For this review, take the finished solid that the model builds, in its own axes (mm). A direction names the side the tool comes from. Round coordinates to 2 decimals unless told otherwise and drop trailing zeros. Loops run counter-clockwise (first coordinate to the right, second up) from the corner with the lowest first, then second, coordinate; pieces in that order, holes last. Notation, with made-up numbers: M 76.25,-39.5 L 85.25,-39.5 A15 ccw 85.25,-17.5 Z; hole C 39.25,42 d6. An arc over 180 degrees is marked long. Write item = value, one per line. Start each with the question number.
```python
from build123d import *

# Parameters (mm, degrees)
SKETCH1_W          = 101.6
SKETCH1_H          = 101.6
EXTRUDE1_DEPTH     = 79.502
SKETCH2_R          = 33.401
EXTRUDE2_DEPTH     = 9.398
CHAMFER1_SIZE      = 1.524
SKETCH3_R          = 13.4874
CUT_EXTRUDE1_DEPTH = 89.9
EXTRUDE3_DEPTH     = 16.002
CHAMFER2_SIZE      = 25.4
SKETCH8_R          = 5.5499
CUT_EXTRUDE3_DEPTH = 12.7


with BuildPart() as part:
    # Sketch1 → Extrude1 (new body)
    with BuildSketch(Plane(origin=(0, 0, 0), x_dir=(1, 0, 0), z_dir=(0, 1, 0))):
        Rectangle(SKETCH1_W, SKETCH1_H)
    extrude(amount=EXTRUDE1_DEPTH)

    # Sketch2 → Extrude2 (add)
    with BuildSketch(Plane(origin=(0, 79.502, 0), x_dir=(-1, 0, 0), z_dir=(0, 1, 0))):
        with Locations(Location((0, 0, 0), (0, 0, 90))):  # turned: the seam where the file's is
            Circle(SKETCH2_R)
    extrude(amount=EXTRUDE2_DEPTH)

    # Chamfer1
    chamfer1_edges = [part.edges().sort_by_distance(p)[0] for p in [
        (0, 88.9, -33.401),
    ]]
    chamfer(chamfer1_edges, length=CHAMFER1_SIZE)

    # Sketch3 → Cut-Extrude1 (cut, through all)
    with BuildSketch(Plane(origin=(0, 88.9, 0), x_dir=(1, 0, 0), z_dir=(0, 1, 0))):
        with Locations(Location((0, 0, 0), (0, 0, 270))):  # turned: the seam where the file's is
            Circle(SKETCH3_R)
    extrude(amount=-CUT_EXTRUDE1_DEPTH, mode=Mode.SUBTRACT)

    # Sketch7 → Extrude3 (add)
    with BuildSketch(Plane.XZ):
        with BuildLine():
            Line((50.8, 50.8), (82.55, 50.8))
            Line((82.55, 50.8), (82.55, 6.731))
            Line((82.55, 6.731), (63.5, 6.731))
            ThreePointArc((63.5, 6.731), (56.769, 0), (63.5, -6.731))
            Line((63.5, -6.731), (82.55, -6.731))
            Line((82.55, -6.731), (82.55, -50.8))
            Line((82.55, -50.8), (50.8, -50.8))
            Line((50.8, -50.8), (50.8, 50.8))
        make_face()
        with BuildLine():
            Line((-82.55, -6.731), (-82.55, -50.8))
            Line((-82.55, -50.8), (-50.8, -50.8))
            Line((-50.8, -50.8), (-50.8, 50.8))
            Line((-50.8, 50.8), (-82.55, 50.8))
            Line((-82.55, 50.8), (-82.55, 6.731))
            Line((-82.55, 6.731), (-63.5, 6.731))
            ThreePointArc((-63.5, 6.731), (-56.769, 0), (-63.5, -6.731))
            Line((-63.5, -6.731), (-82.55, -6.731))
        make_face()
    extrude(amount=-EXTRUDE3_DEPTH)

    # Chamfer2
    chamfer2_edges = [part.edges().sort_by_distance(p)[0] for p in [
        (-82.55, 8.001, -50.8),
        (82.55, 8.001, -50.8),
        (82.55, 8.001, 50.8),
        (-82.55, 8.001, 50.8),
    ]]
    chamfer(chamfer2_edges, length=CHAMFER2_SIZE)

    # Sketch8 → Cut-Extrude3 (cut)
    with BuildSketch(Plane.XY.offset(50.8)):
        with Locations((0, 69.85)):
            Circle(SKETCH8_R)
        with Locations((0, 12.7)):
            Circle(SKETCH8_R)
    extrude(amount=-CUT_EXTRUDE3_DEPTH, mode=Mode.SUBTRACT)


solid = part.part
```
(1) Add section D-D on z = -40.5. Write out the cut boundary in (x, y), and give its area (3 significant figures).
(2) Wall thickness on L1, parallel to Y at x = 0, z = 47.5; L2, parallel to X at y = 64, z = 17; L3, parallel to Z at x = 8.5, y = 76: over which ranges is each line inside the solid? List them lowest first.
(3) Tool access review of faces 4 (the flat face through (-1, 79.502, -35)), 5 (the flat face through (-50.8, 47, 1)), 6 (the flat face through (-73, 8, -6.731)), 7 (the flat face through (0, 13, 38.1)): name each direction out of +Z, -Z, +X, -X, +Y, -Y from which nothing blocks a thin tool from reaching the whole face with its end or side.
(4) Add section A-A on x = -67.5. Write out the cut boundary in (y, z), and give its area (3 significant figures).
(5) Add section B-B on y = 12.7. Write out the cut boundary in (x, z), and give its area (3 significant figures).
(6) For pin 1 Ø8 at (x, y) = (70, 6) entering from -Z; pin 2 Ø8 at (x, y) = (72.5, 6.5) entering from +Z; pin 3 Ø10 at (x, z) = (-60, 21) entering from +Y, all flat-tipped, find the tip position at first contact; note any pin that passes through.
(7) Add section C-C on z = 41. Write out the cut boundary in (x, y), and give its area (3 significant figures).
(8) Draft analysis for pull direction Z (two halves, no side actions). For faces 1 (the flat face through (73, 8, -6.731)), 2 (the flat face through (-70.03, 7.89, -37.92)), 3 (the flat face through (50.8, 47, 1)), state which applies: +Z half, -Z half, draft (parallel to the pull), parting line (faces both ways), or undercut.
Answer sheet:
q1.outline = M -67.45,0 L 67.45,0 L 67.45,16 L 50.8,16 L 50.8,79.5 L -50.8,79.5 L -50.8,16 L -67.45,16 Z
q1.area = 8,610 mm²
q2.L1 = 0 to 7.15, 18.25 to 64.3, 75.4 to 79.5
q2.L2 = -50.8 to 50.8
q2.L3 = -50.8 to -10.47, 10.47 to 50.8
q3.face_4 = +Y
q3.face_5 = +Z, -Z, -X, +Y
q3.face_6 = -X, +Y, -Y
q3.face_7 = +Z
q4.outline = M 0,-40.45 L 16,-40.45 L 16,-6.73 L 0,-6.73 Z; M 0,6.73 L 16,6.73 L 16,40.45 L 0,40.45 Z
q4.area = 1,080 mm²
q5.outline = M -82.55,-25.4 L -57.15,-50.8 L 57.15,-50.8 L 82.55,-25.4 L 82.55,-6.73 L 63.5,-6.73 A6.73 cw 63.5,6.73 L 82.55,6.73 L 82.55,25.4 L 57.15,50.8 L 5.55,50.8 L 5.55,38.1 L -5.55,38.1 L -5.55,50.8 L -57.15,50.8 L -82.55,25.4 L -82.55,6.73 L -63.5,6.73 A6.73 cw -63.5,-6.73 L -82.55,-6.73 Z; hole C 0,0 d26.97
q5.area = 14,100 mm²
q6.pin_1 = -41.95
q6.pin_2 = 39.45
q6.pin_3 = 16
q7.outline = M -66.95,0 L 66.95,0 L 66.95,16 L 50.8,16 L 50.8,79.5 L -50.8,79.5 L -50.8,16 L -66.95,16 Z; hole C 0,12.7 d11.1; hole C 0,69.85 d11.1
q7.area = 8,400 mm²
q8.face_1 = undercut
q8.face_2 = -Z half
q8.face_3 = draft
